Here's the drawing with two shaded views (mm, measured from the low corner). I have some questions. A direction names the side the tool comes from. Coordinates: 2 decimals unless noted, no trailing zeros. Order: outer loops, then holes, each group sorted by start corner. A loop starts at its lowest first (then second) coordinate and runs counter-clockwise, first axis right, second up. Notation, with made-up numbers: (-4.75, 16) -> (11.25, 16) arc R13 ccw to (11.25, 32) -> close; hole circle Ø9 at (-37.75, 80). An arc over 180 degrees is marked (long way). Answer in a Markdown table with one row per item. Add a question column.
1. On a 3-axis mill with a long thin cutter (end or side, diameter ignored), from which of +Z, -Z, +X, -X, +Y, -Y can I reach the whole of each face in a straight line? I mean the marked faces 5, 6 and 7. Say none if no direction works.
2. We'd pull the mould along X, two halves only. Please class the marked faces 1, 2, 3 and 4: pulls with the +X half, pulls with the -X half, needs draft (parallel to the pull), parting line crosses it, or undercut.
3. Imagine slicing it at B-B on z = 47.5. Write out the boundary of the cut face in (x, y), plus the area to 3 significant figures.
4. Imagine slicing it at C-C on y = 10.5. Write out the boundary of the cut face in (x, z).
5. Will this pin go through, and if not, where does the flat tip stop? pin 1 (1.5 mm diameter, centred on x = 14, y = 5.5, fed in from -Z).
6. Imagine slicing it at A-A on y = 1.25. Write out the boundary of the cut face in (x, z).
7. Imagine slicing it at D-D on y = 5.5. Write out the boundary of the cut face in (x, z).
8. If I drill on line 1 along X through (y, z) = (4.5, 38); line 2 along Y through (x, z) = (20.25, 10.5); line 3 along Y through (x, z) = (11.25, 46), over which ranges is the centre line in solid material (lowest first)? Write a range as [from, to].
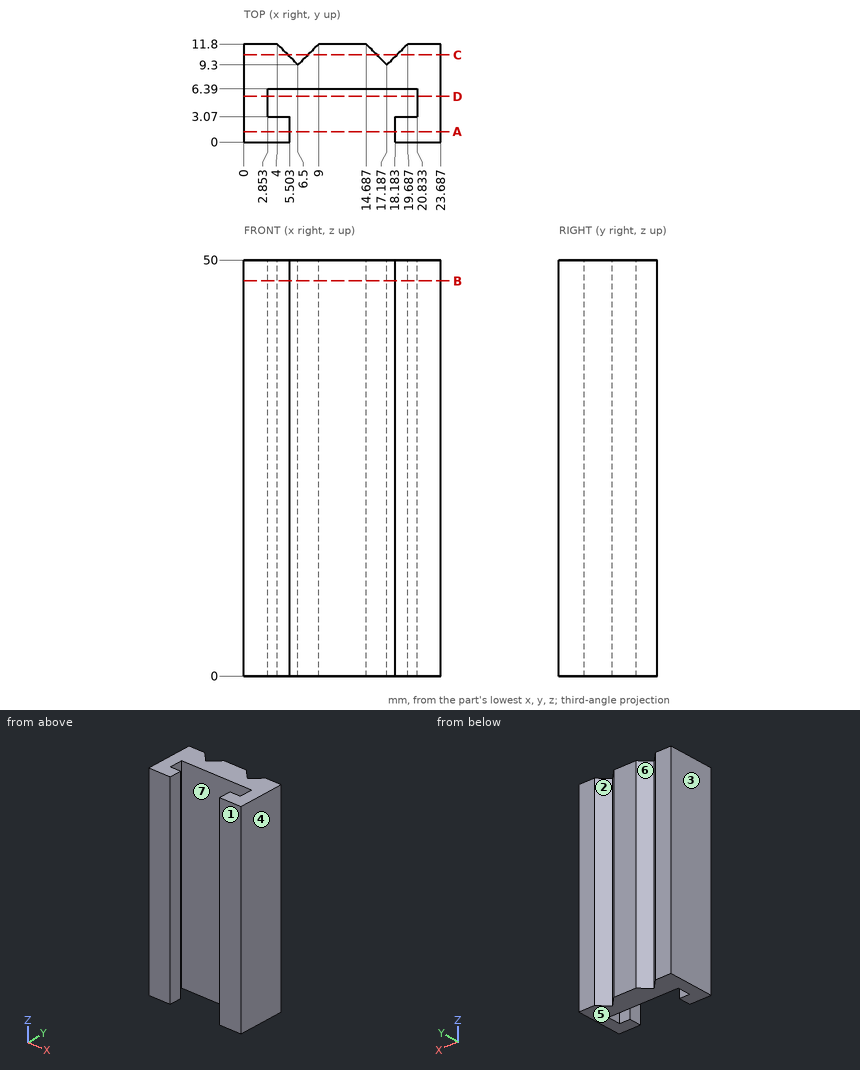
Answers follow:
| question | item | result |
|---|---|---|
| 1 | face 5 | -Z, +X, -X, +Y, -Y |
| 1 | face 6 | +Z, -Z, +Y |
| 1 | face 7 | +Z, -Z |
| 2 | face 1 | needs draft |
| 2 | face 2 | undercut |
| 2 | face 3 | pulls with the -X half |
| 2 | face 4 | pulls with the +X half |
| 3 | outline | (0, 0) -> (5.5, 0) -> (5.5, 3.07) -> (2.85, 3.07) -> (2.85, 6.39) -> (20.83, 6.39) -> (20.83, 3.07) -> (18.18, 3.07) -> (18.18, 0) -> (23.69, 0) -> (23.69, 11.8) -> (19.69, 11.8) -> (17.19, 9.3) -> (14.69, 11.8) -> (9, 11.8) -> (6.5, 9.3) -> (4, 11.8) -> (0, 11.8) -> close |
| 3 | area | 168 mm² |
| 4 | outline | (0, 0) -> (5.3, 0) -> (5.3, 50) -> (0, 50) -> close; (7.7, 0) -> (15.99, 0) -> (15.99, 50) -> (7.7, 50) -> close; (18.39, 0) -> (23.69, 0) -> (23.69, 50) -> (18.39, 50) -> close |
| 5 | pin 1 | passes through |
| 6 | outline | (0, 0) -> (5.5, 0) -> (5.5, 50) -> (0, 50) -> close; (18.18, 0) -> (23.69, 0) -> (23.69, 50) -> (18.18, 50) -> close |
| 7 | outline | (0, 0) -> (2.85, 0) -> (2.85, 50) -> (0, 50) -> close; (20.83, 0) -> (23.69, 0) -> (23.69, 50) -> (20.83, 50) -> close |
| 8 | line 1 | x = [0, 2.85], [20.83, 23.69] |
| 8 | line 2 | y = [0, 3.07], [6.39, 11.8] |
| 8 | line 3 | y = [6.39, 11.8] |
